Build history of the part. All positions in model axes, mm. Coordinates: 2 decimals unless noted, no trailing zeros. Loops run counter-clockwise (first coordinate to the right, second up) from the corner with the lowest first, then second, coordinate; pieces in that order, holes last.
(1) Two-plate mould, pull along Z, no slides. Class faces 1 (the face through (1, -3.175, 0)), 2 (the face through (-12.766, -0.685, -14.834)), 3 (the face through (-1, 0, -33.655)), 4 (the face through (0, 0, 33.655)): pulls with the +Z half, pulls with the -Z half, needs draft (parallel to the pull), parting line crosses it, or undercut.
(2) Wall check: L1, parallel to X at y = 1.75, z = -27.5; L2, parallel to Z at x = 50.8, y = -1.55 (3 decimals); L3, parallel to X at y = 2.5, z = 13. Give the ranges that are in metal, low to high.
(3) Slice it at C-C (x = -35). Give the cut face in (y, z) (3 decimals), and give its area (3 significant figures).
(4) Slice it at B-B (x = -50.8). Give the cut face in (y, z) (3 decimals).
(5) Slice it at A-A (x = -12.7). Give the cut face in (y, z) (3 decimals), and give its area (3 significant figures).
(6) Flat gauge pins, fed straight in: P1, Ø4, axis at x = -27.78, z = 23.4, coming from the -Y side; P2, Ø2.5, axis at x = 27.77, z = 23.4, coming from the +Y side; P3, Ø2, axis at x = 50, z = -14, coming from the +Y side; P4, Ø5, axis at x = -12.7, z = 13.335, coming from the +Y side (3 decimals). Where does each tip first touch, or does it go through?
Autodesk Inventor part; units mm, degrees
ref_plane "YZ Plane" through (0, 0, 0) normal (1, 0, 0) x (0, 1, 0)
ref_plane "XZ Plane" through (0, 0, 0) normal (0, 1, 0) x (-1, 0, 0)
ref_plane "XY Plane" through (0, 0, 0) normal (0, 0, 1) x (1, 0, 0)
sketch "Sketch1" plane through (0, 0, 0) normal (0, 1, 0) x (-1, 0, 0)
  line L0 (-63.5, 33.655) -> (63.5, 33.655)
  line L1 (63.5, 33.655) -> (63.5, -33.655)
  line L2 (63.5, -33.655) -> (-63.5, -33.655)
  line L3 (-63.5, -33.655) -> (-63.5, 33.655)
  line L4 (-63.5, 33.655) -> (63.5, -33.655) construction
  line L5 (63.5, 33.655) -> (-63.5, -33.655) construction
  point P0 (0, 0)
  dimension "d0" = 127
  dimension "d1" = 67.31
extrude "Extrusion1" add sketch "Sketch1" along normal mid plane 6.35
sketch "Sketch4" plane through (0, 3.175, 0) normal (0, 1, 0) x (1, 0, 0)
  line L0 (63.5, 33.655) -> (-63.5, 33.655)
  line L1 (-63.5, -33.655) -> (63.5, -33.655)
  line L2 (-63.5, 33.655) -> (-63.5, -33.655)
  line L3 (63.5, -33.655) -> (63.5, 33.655)
  point P0 (0, 0)
  point P1 (-50.8, 13.335)
  point P2 (-50.8, -13.335)
  point P3 (-12.7, 13.335)
  point P4 (-12.7, -13.335)
  point P5 (12.7, 13.335)
  point P6 (12.7, -13.335)
  point P7 (50.8, 13.335)
  point P8 (50.8, -13.335)
  point P9 (-50.8, -33.655)
  point P10 (50.8, -33.655)
  point P11 (-63.5, -20.955)
  point P12 (63.5, -20.955)
  dimension "d24" = 20.32
  dimension "d25" = 20.32
  dimension "d26" = 12.7
  dimension "d27" = 12.7
  dimension "d28" = 50.8
  dimension "d29" = 50.8
hole "Hole2" at (-50.8, 3.175, -13.335) at (-50.8, 3.175, 13.335) at (-12.7, 3.175, -13.335) at (-12.7, 3.175, 13.335) at (12.7, 3.175, -13.335) at (12.7, 3.175, 13.335) at (50.8, 3.175, -13.335) at (50.8, 3.175, 13.335) direction (0, -1, 0) diameter 3 depth 25.4 tip angle 118 countersink diameter 5.6 countersink angle 90
chamfer "Chamfer1" distance 19.05 angle 60 1 edges at (-63.5, 0, 33.655) measured on face at (-63.5, -1.0583, 11.2183)
sketch "Sketch5" plane through (0, -3.175, 0) normal (0, -1, 0) x (1, 0, 0)
  circle A0 centre (-27.7751, 23.3958) radius 1.7018
  circle A1 centre (27.7749, 23.3958) radius 1.7018
  circle A2 centre (27.7749, -27.4042) radius 1.7018
  circle A3 centre (-27.7751, -27.4042) radius 1.7018
  point P0 (0, 0)
hole "Hole3" at (-27.7751, -3.175, 23.3958) at (27.7749, -3.175, 23.3958) at (27.7749, -3.175, -27.4042) at (-27.7751, -3.175, -27.4042) direction (0, 1, 0) diameter 3.4036 end through all countersink diameter 6.2992 countersink angle 90
chamfer "Chamfer2" distance 19.05 angle 60 1 edges at (63.5, 0, 33.655) measured on face at (63.5, 1.0583, 11.2183)
properties part number "DPLX_P035 Spark Gap Shielding Middle" material "Polyethylene, High Density"
Response values:
1. face 1: needs draft
1. face 2: undercut
1. face 3: pulls with the -Z half
1. face 4: pulls with the +Z half
2. L1: x = -63.5 to -29.47, -26.08 to 26.08, 29.47 to 63.5
2. L2: z = -33.655 to -14.835, -11.835 to 11.835, 14.835 to 21.937
2. L3: x = -63.5 to -52.9, -48.7 to -14.8, -10.6 to 10.6, 14.8 to 48.7, 52.9 to 63.5
3. outline: (-3.175, -33.655) - (3.175, -33.655) - (3.175, 31.059) - (-3.175, 31.059) - close
3. area: 411 mm2
4. outline: (-3.175, -33.655) - (3.175, -33.655) - (3.175, -16.135) - (1.875, -14.835) - (-3.175, -14.835) - close; (-3.175, -11.835) - (1.875, -11.835) - (3.175, -10.535) - (3.175, 10.535) - (1.875, 11.835) - (-3.175, 11.835) - close; (-3.175, 14.835) - (1.875, 14.835) - (3.175, 16.135) - (3.175, 21.937) - (-3.175, 21.937) - close
5. outline: (-3.175, -33.655) - (3.175, -33.655) - (3.175, -16.135) - (1.875, -14.835) - (-3.175, -14.835) - close; (-3.175, -11.835) - (1.875, -11.835) - (3.175, -10.535) - (3.175, 10.535) - (1.875, 11.835) - (-3.175, 11.835) - close; (-3.175, 14.835) - (1.875, 14.835) - (3.175, 16.135) - (3.175, 33.655) - (-3.175, 33.655) - close
5. area: 386 mm2
6. P1: stops at y = -2.03
6. P2: passes through
6. P3: stops at y = 2.42
6. P4: stops at y = 2.875
